```python
from build123d import *

# Parameters (mm, degrees)
SKETCH049_W             = 34
SKETCH049_H             = 37.5
PAD032_DEPTH            = 6
SKETCH050_W             = 30
SKETCH050_H             = 33.5
POCKET014_DEPTH         = 4
SKETCH051_W             = 26
SKETCH051_H             = 29.5
POCKET015_DEPTH         = 2.001
SKETCH052_W             = 4
SKETCH052_H             = 28
POCKET016_DEPTH         = 6.001
REVOLUTION_ANGLE        = 180
REVOLUTION001_ANGLE     = -180
REVOLUTION002_ANGLE     = 180
BODY009_PLACEMENT_ANGLE = -90


with BuildPart() as part:
    # Sketch049 → Pad032 (new body)
    with BuildSketch(Plane.XY):
        with Locations((17, 18.75)):
            Rectangle(SKETCH049_W, SKETCH049_H)
    extrude(amount=PAD032_DEPTH)

    # Sketch050 (on Face6 of Pad032) → Pocket014 (cut)
    with BuildSketch(Plane.XY.offset(6)):
        with Locations((17, 18.75)):
            Rectangle(SKETCH050_W, SKETCH050_H)
    extrude(amount=-POCKET014_DEPTH, mode=Mode.SUBTRACT)

    # Sketch051 (on Face11 of Pocket014) → Pocket015 (cut, through all)
    with BuildSketch(Plane.XY.offset(2)):
        with Locations((17, 18.75)):
            Rectangle(SKETCH051_W, SKETCH051_H)
    extrude(amount=-POCKET015_DEPTH, mode=Mode.SUBTRACT)

    # Sketch052 (on Face5 of Pocket015) → Pocket016 (cut, through all)
    with BuildSketch(Plane.XY.offset(6)):
        with Locations((2, 18.75)):
            Rectangle(SKETCH052_W, SKETCH052_H)
    extrude(amount=-POCKET016_DEPTH, mode=Mode.SUBTRACT)

    # Sketch053 (on Face17 of Pocket016) → Revolution (revolve)
    with BuildSketch(Plane(origin=(32, 0, 0), x_dir=(0, -1, 0), z_dir=(-1, 0, 0))):
        with BuildLine():
            ThreePointArc((-28.5, 5), (-29.5, 6), (-30.5, 5))
            Line((-28.5, 5), (-30.5, 5))
        make_face()
        with BuildLine():
            ThreePointArc((-7, 5), (-8, 6), (-9, 5))
            Line((-9, 5), (-7, 5))
        make_face()
    revolve(axis=Axis((32, 29.201832, 5), (0, -1, 0)), revolution_arc=REVOLUTION_ANGLE)

    # Sketch054 (on Face16 of Revolution) → Revolution001 (revolve)
    with BuildSketch(Plane(origin=(0, 2, 0), x_dir=(-1, 0, 0), z_dir=(0, 1, 0))):
        with BuildLine():
            ThreePointArc((-3, 5), (-4, 6), (-5, 5))
            Line((-5, 5), (-3, 5))
        make_face()
    revolve(axis=Axis((5, 2, 5), (1, 0, 0)), revolution_arc=REVOLUTION001_ANGLE)

    # Sketch055 (on Face19 of Revolution001) → Revolution002 (revolve)
    with BuildSketch(Plane.XZ.offset(-35.5)):
        with BuildLine():
            ThreePointArc((5, 5), (4, 6), (3, 5))
            Line((3, 5), (5, 5))
        make_face()
    revolve(axis=Axis((5, 35.5, 5), (1, 0, 0)), revolution_arc=REVOLUTION002_ANGLE)


with BuildPart() as part_1:
    # Body009 placement: moved
    add(part.part.moved(Location((5, 40, 105.27))).rotate(Axis((5, 40, 105.27), (0, 0, 1)), BODY009_PLACEMENT_ANGLE))


solid = part_1.part
```
Geometry check sheet. Reference: the model listing, model coordinates, mm. A direction names the side the tool comes from. Coordinates: 2 decimals unless noted, no trailing zeros. Order: outer loops, then holes, each group sorted by start corner. A loop starts at its lowest first (then second) coordinate and runs counter-clockwise, first axis right, second up.
Item 1: Scan lines: line 1 along X through (y, z) = (35.5, 106.6); line 2 along X through (y, z) = (8.5, 109.65); line 3 along X through (y, z) = (22, 111.05). Record each from-to range of solid material in increasing order.
Item 2: Tool access check on faces 4 (the flat face through (9.75, 38.5, 107.6)), 5 (the flat face through (38.5, 23, 106)), 6 (the flat face through (23, 6, 108)), 7 (the flat face through (8, 38, 109)), 8 (the flat face through (5, 23, 108)). Record the directions out of +Z, -Z, +X, -X, +Y, -Y that give a thin tool (end or side, any length) a straight path to the whole face; none if there is none.
Item 3: Section check C-C (z = 108.7). Enter the section's corners in (x, y), plus the area to 3 significant figures.
Item 4: Section check D-D (x = 27). Enter the section's corners in (y, z), plus the area to 3 significant figures.
Item 5: Depth check by flat-ended pin: pin 1 (2 mm diameter, centred on x = 18.5, z = 106, fed in from +Y). Enter the tip coordinate at first touch or a pass-through.
Item 6: Section check B-B (x = 8.5). Enter the section's corners in (y, z).
Item 7: Mould release check, pull along X, two halves, no side actions. Record for faces 1 (the flat face through (37.75, 38.5, 107.6)), 2 (the flat face through (42.5, 23, 108)), 3 (the flat face through (22, 9, 105.27)): released by +X, released by -X, zero draft, split by the parting line, or undercut.
Item 8: Section check A-A (y = 30.5). Enter the section's corners in (x, z), plus the area to 3 significant figures.
Check sheet entries:
1. line 1: x = 5 to 9, 38.5 to 42.5
1. line 2: x = 5 to 7, 12.4 to 13.6, 33.9 to 35.1, 40.5 to 42.5
1. line 3: x = 5 to 7, 40.5 to 42.5
2. face 4: +Z, -Z, +Y
2. face 5: +Z, -Z
2. face 6: +Z, -Z, +X, -X, -Y
2. face 7: +Z
2. face 8: +Z, -Z, -X, +Y, -Y
3. outline: (5, 6) - (42.5, 6) - (42.5, 40) - (37.75, 40) - (37.75, 38) - (40.5, 38) - (40.5, 8) - (7, 8) - (7, 38) - (9.75, 38) - (9.75, 40) - (5, 40) - close
3. area: 214 mm2
4. outline: (6, 105.27) - (10, 105.27) - (10, 107.27) - (8, 107.27) - (8, 111.27) - (6, 111.27) - close
4. area: 16.0 mm2
5. pin 1: stops at y = 10
6. outline: (6, 105.27) - (40, 105.27) - (40, 111.27) - (38, 111.27) - (38, 107.27) - (8, 107.27) - (8, 111.27) - (6, 111.27) - close
7. face 1: undercut
7. face 2: released by +X
7. face 3: zero draft
8. outline: (5, 105.27) - (9, 105.27) - (9, 107.27) - (7, 107.27) - (7, 111.27) - (5, 111.27) - close; (38.5, 105.27) - (42.5, 105.27) - (42.5, 111.27) - (40.5, 111.27) - (40.5, 107.27) - (38.5, 107.27) - close
8. area: 32.0 mm2
